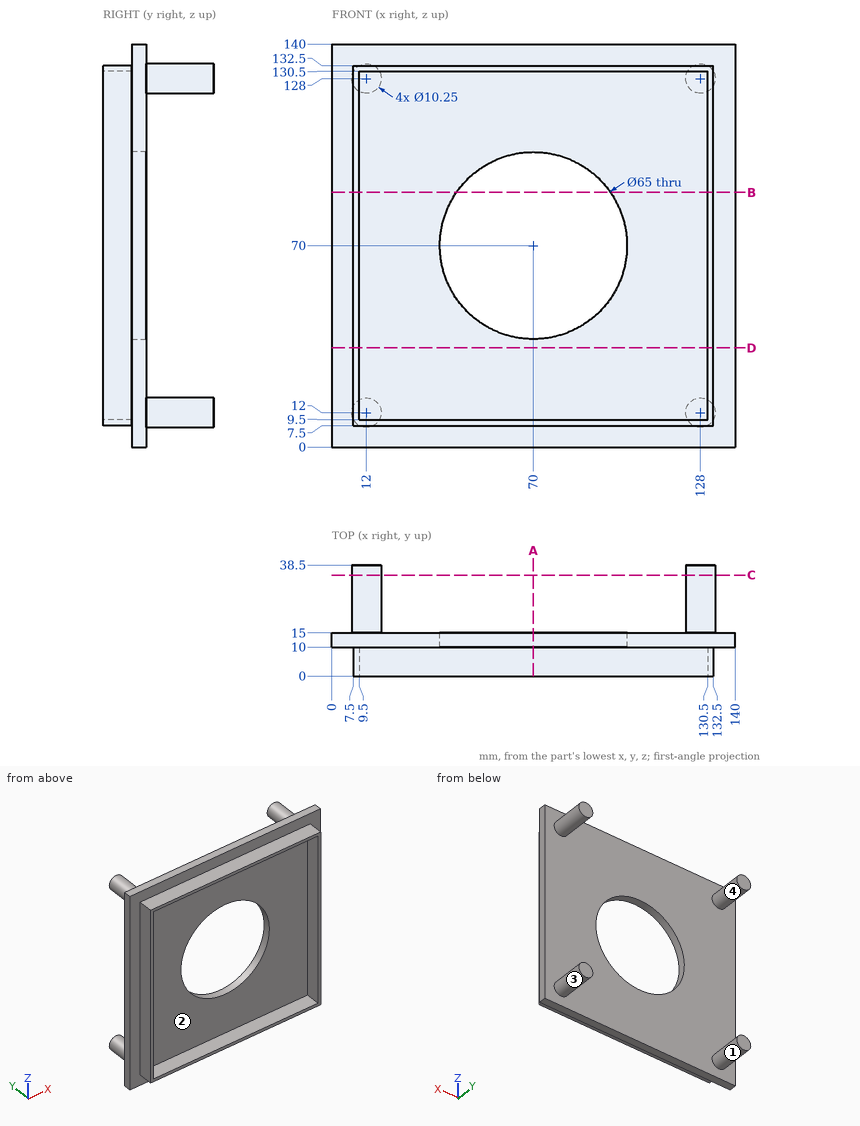
Source: three-view drawing plus pictorial views. Frame: mm from the lowest corner of the part. A direction names the side the tool comes from. Round coordinates to 2 decimals unless told otherwise and drop trailing zeros. Loops run counter-clockwise (first coordinate to the right, second up) from the corner with the lowest first, then second, coordinate; pieces in that order, holes last. Notation, with made-up numbers: (-35.75, -24) -> (-30.75, -24) arc R27 cw to (-30.75, -7) -> close; hole circle Ø7 at (76.5, -15.5). An arc over 180 degrees is marked (long way). Use one line per item in the form item = value.
Item 1: Draft query along Z for the marked faces 3 and 4. Return one class per face: released by +Z, released by -Z, zero draft, split by the parting line, or undercut.
Evaluation:
face_3 = undercut
face_4 = undercut
Item 2: Material intervals for probe 1 along X at (y, z) = (6, 36.5); probe 2 along X at (y, z) = (11, 70), sorted ascending.
Evaluation:
probe_1 = 7.5 to 9.5, 130.5 to 132.5
probe_2 = 0 to 37.5, 102.5 to 140
Item 3: Contact query for flat-ended pins moving along their axis: pin 1 Ø11 at (y, z) = (2.5, 47) entering from -X; pin 2 Ø5 at (x, y) = (89.5, 7) entering from +Z; pin 3 Ø8 at (x, z) = (108.5, 22) entering from +Y; pin 4 Ø10 at (y, z) = (7.5, 114.5) entering from -X. Output: stop coordinate, or through.
Evaluation:
pin_1 = 7.5
pin_2 = 132.5
pin_3 = 15
pin_4 = 0
Item 4: Cut plane B-B on z = 88.5. Output: boundary loops of the cut face in (x, y).
Evaluation:
outline = (0, 10) -> (7.5, 10) -> (7.5, 0) -> (9.5, 0) -> (9.5, 10) -> (43.28, 10) -> (43.28, 15) -> (0, 15) -> close; (96.72, 10) -> (130.5, 10) -> (130.5, 0) -> (132.5, 0) -> (132.5, 10) -> (140, 10) -> (140, 15) -> (96.72, 15) -> close
Item 5: Access query for the marked faces 1 and 2. Directions: +Z, -Z, +X, -X, +Y, -Y. A direction counts if a zero-diameter tool reaches every point of the face in a straight line with its end or side. Return the directions, or none.
Evaluation:
face_1 = +Y
face_2 = -Y
Item 6: Cut plane C-C on y = 35. Output: boundary loops of the cut face in (x, z) (3 decimals).
Evaluation:
outline = circle Ø10.25 at (12, 12); circle Ø10.25 at (12, 128); circle Ø10.25 at (128, 12); circle Ø10.25 at (128, 128)
Item 7: Cut plane A-A on x = 70. Output: boundary loops of the cut face in (y, z).
Evaluation:
outline = (0, 7.5) -> (10, 7.5) -> (10, 0) -> (15, 0) -> (15, 37.5) -> (10, 37.5) -> (10, 9.5) -> (0, 9.5) -> close; (0, 130.5) -> (10, 130.5) -> (10, 102.5) -> (15, 102.5) -> (15, 140) -> (10, 140) -> (10, 132.5) -> (0, 132.5) -> close
Item 8: Cut plane D-D on z = 34.5. Output: boundary loops of the cut face in (x, y).
Evaluation:
outline = (0, 10) -> (7.5, 10) -> (7.5, 0) -> (9.5, 0) -> (9.5, 10) -> (130.5, 10) -> (130.5, 0) -> (132.5, 0) -> (132.5, 10) -> (140, 10) -> (140, 15) -> (0, 15) -> close
